from build123d import *
from OCP.BRepFilletAPI import BRepFilletAPI_MakeChamfer

# Parameters (mm, degrees)
SKETCH1_W                 = 148
SKETCH1_H                 = 12.7
BOSS_EXTRUDE1_DEPTH       = 25.4
CHAMFER1_SIZE             = 8
CHAMFER1_SIZE2            = 50
M5X0_8_TAPPED_HOLE1_D     = 4.2
M5X0_8_TAPPED_HOLE1_DEPTH = 12
M5X0_8_TAPPED_HOLE1_TIP   = 1.2618073
FILLET1_R                 = 10


with BuildPart() as part:
    # Sketch1 → Boss-Extrude1 (new body)
    with BuildSketch(Plane(origin=(0, 0, 0), x_dir=(1, 0, 0), z_dir=(0, 1, 0))):
        Rectangle(SKETCH1_W, SKETCH1_H)
    extrude(amount=BOSS_EXTRUDE1_DEPTH)

    # Chamfer1: one chamfer whose edges measure the first distance from different faces: ONE call of the kernel's chamfer builder (chamfer() names one face for all edges)
    chamfer1_edges_1 = [part.edges().sort_by_distance(p)[0] for p in [
        (-74, 25.4, 0),
    ]]
    chamfer1_side_1 = [part.faces().sort_by_distance(p)[0] for p in [
        (-74, 12.7, 0),
    ]]
    chamfer1_edges_2 = [part.edges().sort_by_distance(p)[0] for p in [
        (74, 25.4, 0),
    ]]
    chamfer1_side_2 = [part.faces().sort_by_distance(p)[0] for p in [
        (74, 12.7, 0),
    ]]
    chamfer1 = BRepFilletAPI_MakeChamfer(part.part.solid().wrapped)
    for e in chamfer1_edges_1:
        chamfer1.Add(CHAMFER1_SIZE, CHAMFER1_SIZE2, e.wrapped, chamfer1_side_1[0].wrapped)  # the first distance lies on this face
    for e in chamfer1_edges_2:
        chamfer1.Add(CHAMFER1_SIZE, CHAMFER1_SIZE2, e.wrapped, chamfer1_side_2[0].wrapped)  # the first distance lies on this face
    add(Compound.cast(chamfer1.Shape()), mode=Mode.REPLACE)

    # M5x0.8 Tapped Hole1
    with Locations(Plane(origin=(0, 0, 0), x_dir=(-1, 0, 0), z_dir=(0, -1, 0))):
        with Locations((66, 0), (22, 0), (-22, 0), (-66, 0)):
            Hole(M5X0_8_TAPPED_HOLE1_D / 2, depth=M5X0_8_TAPPED_HOLE1_DEPTH)
            with Locations((0, 0, -(M5X0_8_TAPPED_HOLE1_DEPTH + M5X0_8_TAPPED_HOLE1_TIP / 2))):  # 118° drill point
                Cone(0, M5X0_8_TAPPED_HOLE1_D / 2, M5X0_8_TAPPED_HOLE1_TIP, mode=Mode.SUBTRACT)

    # Fillet1
    fillet1_edges = [part.edges().sort_by_distance(p)[0] for p in [
        (-24, 25.4, 0),
        (24, 25.4, 0),
        (74, 17.4, 0),
        (-74, 17.4, 0),
    ]]
    fillet(fillet1_edges, radius=FILLET1_R)


solid = part.part
Verification items for the finished model (mm, model axes). A direction names the side the tool comes from. Coordinates: 2 decimals unless noted, no trailing zeros. Loops run counter-clockwise (first coordinate to the right, second up) from the corner with the lowest first, then second, coordinate; pieces in that order, holes last. Notation, with made-up numbers: (57, 46) -> (111, 46) arc R24 ccw to (111, 61) -> close; hole circle Ø8 at (0.25, 17). An arc over 180 degrees is marked (long way). Answer as a JSON object with one key per item and string values. Group by question number.
Item 1: Sectioned sample at A-A on y = 6.25. Record the boundary of the cut face in (x, z), plus the area to 3 significant figures.
Item 2: Tool access check on faces 1 (the cylindrical face through (-64.06, 6.08, 0.8)), 2 (the flat face through (-1, 13, 6.35)). Record the directions out of +Z, -Z, +X, -X, +Y, -Y that give a thin tool (end or side, any length) a straight path to the whole face; none if there is none.
Item 3: Sectioned sample at C-C on x = -40. Record the boundary of the cut face in (y, z), plus the area to 3 significant figures.
Item 4: Depth check by flat-ended pin: pin 1 (6 mm diameter, centred on y = 14.5, z = 3.5, fed in from -X); pin 2 (6.5 mm diameter, centred on x = 66, z = 0, fed in from +Y); pin 3 (4 mm diameter, centred on x = 52.5, z = -2, fed in from +Y). Enter the tip coordinate at first touch or a pass-through.
Item 5: Sectioned sample at D-D on y = 21.75. Record the boundary of the cut face in (x, z).
Item 6: Scan lines: probe 1 along Z at (x, y) = (66, 8); probe 2 along X at (y, z) = (9.75, 1.5); probe 3 along X at (y, z) = (10.25, 0.25). Record each from-to range of solid material in increasing order.
Item 7: Mould release check, pull along Z, two halves, no side actions. Record for faces 3 (the flat face through (-44.897, 22.057, 0.089)), 4 (the conical face through (65.66, 13.04, 0.14)), 5 (the flat face through (-1, 13, -6.35)): +Z half, -Z half, draft (parallel to the pull), parting line (faces both ways), or undercut.
Item 8: Sectioned sample at B-B on z = 4. Record the boundary of the cut face in (x, y).
Evaluation:
{
 "1": {"outline": "(-74, -6.35) -> (74, -6.35) -> (74, 6.35) -> (-74, 6.35) -> close; hole circle Ø4.2 at (-66, 0); hole circle Ø4.2 at (-22, 0); hole circle Ø4.2 at (22, 0); hole circle Ø4.2 at (66, 0)", "area": "1,820 mm²"},
 "2": {"face 1": "-Y", "face 2": "+Z, +X, -X, +Y, -Y"},
 "3": {"outline": "(0, -6.35) -> (22.84, -6.35) -> (22.84, 6.35) -> (0, 6.35) -> close", "area": "290 mm²"},
 "4": {"pin 1": "stops at x = -73.65", "pin 2": "stops at y = 19.2", "pin 3": "stops at y = 21.16"},
 "5": {"outline": "(-46.81, -6.35) -> (46.81, -6.35) -> (46.81, 6.35) -> (-46.81, 6.35) -> close"},
 "6": {"probe 1": "z = -6.35 to -2.1, 2.1 to 6.35", "probe 2": "x = -73.96 to -67.47, -64.53 to -23.47, -20.53 to 20.53, 23.47 to 64.53, 67.47 to 73.96", "probe 3": "x = -73.9 to -68.09, -63.91 to -24.09, -19.91 to 19.91, 24.09 to 63.91, 68.09 to 73.9"},
 "7": {"face 3": "draft", "face 4": "undercut", "face 5": "-Z half"},
 "8": {"outline": "(-74, 0) -> (74, 0) -> (74, 8.87) arc R10 ccw to (65.58, 18.75) -> (24.78, 25.27) arc R10 ccw to (23.21, 25.4) -> (-23.21, 25.4) arc R10 ccw to (-24.78, 25.27) -> (-65.58, 18.75) arc R10 ccw to (-74, 8.87) -> close"}
}
